Verification items for the finished model (mm, model axes). Round coordinates to 2 decimals unless told otherwise and drop trailing zeros. Loops run counter-clockwise (first coordinate to the right, second up) from the corner with the lowest first, then second, coordinate; pieces in that order, holes last. Notation, with made-up numbers: M -24.5,57 L -18.5,57 A17 ccw -18.5,86 Z; hole C 76.5,36 d5. An arc over 180 degrees is marked long. Answer as CSV lines item,"result".
```python
from build123d import *

# Parameters (mm, degrees)
SKETCH1_R           = 4
BOSS_EXTRUDE1_DEPTH = 4
SKETCH2_R           = 2
BOSS_EXTRUDE2_DEPTH = 6
CHAMFER1_SIZE       = 0.25
SKETCH3_R           = 2
BOSS_EXTRUDE3_DEPTH = 3
CHAMFER2_SIZE       = 0.25
FILLET2_R           = 8


with BuildPart() as part:
    # Sketch1 → Boss-Extrude1 (new body)
    with BuildSketch(Plane.XY):
        with BuildLine():
            ThreePointArc((5.656854249, 5.656854249), (0, 8), (-5.656854249, 5.656854249))
            Line((-5.656854249, 5.656854249), (-18.697995031, -7.384286532))
            ThreePointArc((-18.697995031, -7.384286532), (-46.023235671, 1.192804635), (-70.171144566, 16.591303421))
            ThreePointArc((-70.171144566, 16.591303421), (-78.62508069, 15.86263065), (-77.896407918, 7.408694525))
            ThreePointArc((-77.896407918, 7.408694525), (0, -21), (77.896407918, 7.408694525))
            ThreePointArc((77.896407918, 7.408694525), (78.62508069, 15.86263065), (70.171144566, 16.591303421))
            ThreePointArc((70.171144566, 16.591303421), (46.023235671, 1.192804635), (18.697995031, -7.384286532))
            Line((18.697995031, -7.384286532), (5.656854249, 5.656854249))
        make_face()
        Circle(SKETCH1_R, mode=Mode.SUBTRACT)
    extrude(amount=BOSS_EXTRUDE1_DEPTH)

    # Sketch2 → Boss-Extrude2 (add)
    with BuildSketch(Plane.XY.offset(4)):
        with Locations((-74.033776242, 11.999998973)):
            Circle(SKETCH2_R)
    extrude(amount=BOSS_EXTRUDE2_DEPTH)

    # Chamfer1
    chamfer1_edges = [part.edges().sort_by_distance(p)[0] for p in [
        (-76.033776242, 11.999998973, 10),
    ]]
    chamfer(chamfer1_edges, length=CHAMFER1_SIZE)

    # Sketch3 → Boss-Extrude3 (add)
    with BuildSketch(Plane(origin=(0, 0, 0), x_dir=(-1, 0, 0), z_dir=(0, 0, -1))):
        with Locations((-75.321320134, 10.469564157)):
            Circle(SKETCH3_R)
    extrude(amount=BOSS_EXTRUDE3_DEPTH)

    # Chamfer2
    chamfer2_edges = [part.edges().sort_by_distance(p)[0] for p in [
        (77.321320134, 10.469564157, -3),
    ]]
    chamfer(chamfer2_edges, length=CHAMFER2_SIZE)

    # Fillet2
    fillet2_edges = [part.edges().sort_by_distance(p)[0] for p in [
        (18.697995031, -7.384286532, 2),
        (-18.697995031, -7.384286532, 2),
    ]]
    fillet(fillet2_edges, radius=FILLET2_R)


solid = part.part
```
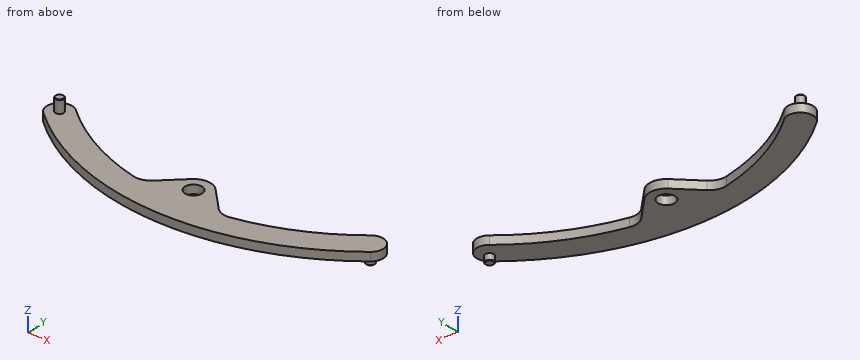
1) Material ranges on probe 1 along Y at (x, z) = (0, 2.1); probe 2 along Z at (x, y) = (36.5, -14.5); probe 3 along Y at (x, z) = (15.5, 3), recorded low to high.
Here are the results:
probe 1,"y = -21 to -4, 4 to 8"
probe 2,"z = 0 to 4"
probe 3,"y = -20 to -4.19"
2) Section check D-D (x = 36.5). Record the cut outline in (y, z).
Here are the results:
outline,"M -15.36,0 L -2.71,0 L -2.71,4 L -15.36,4 Z"
3) Section check A-A (x = 0). Record the cut outline in (y, z), plus the area to 3 significant figures.
Here are the results:
outline,"M -21,0 L -4,0 L -4,4 L -21,4 Z; M 4,0 L 8,0 L 8,4 L 4,4 Z"
area,"84.0 mm^2"
4) Section check B-B (y = 0). Record the cut outline in (x, z).
Here are the results:
outline,"M -68.12,0 L -43.37,0 L -43.37,4 L -68.12,4 Z; M -11.31,0 L -4,0 L -4,4 L -11.31,4 Z; M 4,0 L 11.31,0 L 11.31,4 L 4,4 Z; M 43.37,0 L 68.12,0 L 68.12,4 L 43.37,4 Z"
5) Section check C-C (y = -18). Record the cut outline in (x, z), plus the area to 3 significant figures.
Here are the results:
outline,"M -26.78,0 L 26.78,0 L 26.78,4 L -26.78,4 Z"
area,"214 mm^2"
6) Go/stop test with flat-tipped pins: pin 1 (5 mm diameter, centred on y = 4, z = 5, fed in from +X); pin 2 (11.5 mm diameter, centred on x = -14, y = -3, fed in from -Z); pin 3 (6 mm diameter, centred on y = -7.5, z = 5, fed in from +X). Record where each tip stops, or that it passes through.
Here are the results:
pin 1,"stops at x = 76.55"
pin 2,"stops at z = 0"
pin 3,"stops at x = 60.7"
